Verification items for the finished model (mm, model axes). Face numbers are marked on the shaded views. Round coordinates to 2 decimals unless told otherwise and drop trailing zeros. Loops run counter-clockwise (first coordinate to the right, second up) from the corner with the lowest first, then second, coordinate; pieces in that order, holes last. Notation, with made-up numbers: M 49,19.5 L 59,19.5 A14 ccw 59,34.5 Z; hole C -32.5,-38 d9. An arc over 180 degrees is marked long. Answer as CSV lines item,"result".
Autodesk Inventor part; units mm, degrees
ref_plane "Work Plane1" through (0, 5, 0) normal (0, 1, 0) x (1, 0, 0)
ref_plane "Work Plane2" through (0, 0, 0) normal (0, -1, 0) x (1, 0, 0)
ref_plane "YZ Plane" through (0, 0, 0) normal (1, 0, 0) x (0, 1, 0)
sketch "Sketch1" plane through (0, 0, 0) normal (0, 1, 0) x (-1, 0, 0)
  line L0 (2.8251, -4.9022) -> (-2.8329, -4.8978)
  line L1 (-2.8329, -4.8978) -> (-5.658, 0.0045)
  line L2 (-5.658, 0.0045) -> (-2.8251, 4.9022)
  line L3 (-2.8251, 4.9022) -> (2.8329, 4.8978)
  line L4 (2.8329, 4.8978) -> (5.658, -0.0045)
  line L5 (5.658, -0.0045) -> (2.8251, -4.9022)
  circle A0 centre (0, 0) radius 3
  dimension "d0" = 9.8
  dimension "d1" = 6
extrude "Extrusion1" add sketch "Sketch1" along normal blind 5
fillet "Fillet1" radius 0.8 14 edges at (4.2416, 5, 2.4533) (4.2455, 5, -2.4467) (0.0039, 5, -4.9) (-4.2416, 5, -2.4533) (-4.2455, 5, 2.4467) (-0.0039, 5, 4.9) (-0.0039, 0, 4.9) (4.2416, 0, 2.4533) (4.2455, 0, -2.4467) (0.0039, 0, -4.9) (-4.2416, 0, -2.4533) (-4.2455, 0, 2.4467) (3, 5, 0) (3, 0, 0)
thread "Thread1"
ref_plane "Work Plane1" through (0, 5, 0) normal (0, 1, 0) x (1, 0, 0)
ref_plane "Work Plane2" through (0, 0, 0) normal (0, -1, 0) x (1, 0, 0)
properties part number "m6nut"
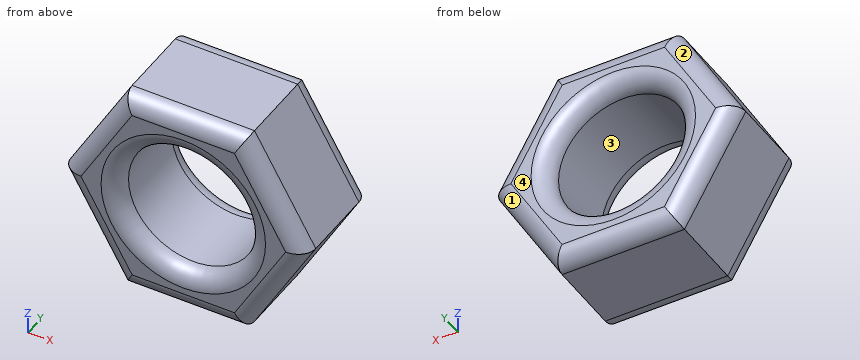
1) Section check A-A (y = 2.8). Record the cut outline in (x, z).
Here are the results:
outline,"M -5.66,0 L -2.83,-4.9 L 2.83,-4.9 L 5.66,0 L 2.83,4.9 L -2.83,4.9 Z; hole C 0,0 d6"
2) Go/stop test with flat-tipped pins: pin 1 (2 mm diameter, centred on y = 1, z = -3.5, fed in from -X); pin 2 (5.5 mm diameter, centred on x = 0, z = 0, fed in from +Y); pin 3 (1 mm diameter, centred on x = 4, z = -0.5, fed in from -Y); pin 4 (1 mm diameter, centred on x = -1, y = 1.5, fed in from +Z). Record where each tip stops, or that it passes through.
Here are the results:
pin 1,"stops at x = -4.21"
pin 2,"passes through"
pin 3,"stops at y = 0"
pin 4,"stops at z = 4.9"
3) Section check B-B (y = 0.5). Record the cut outline in (x, z).
Here are the results:
outline,"M -5.59,0 L -2.79,-4.84 L 2.8,-4.84 L 5.59,0 L 2.79,4.84 L -2.8,4.84 Z; hole C 0,0 d6.12"
4) Draft check along Z on the marked faces 1, 2, 3 and 4. Enter one of: +Z half, -Z half, draft (parallel to the pull), parting line (faces both ways), or undercut.
Here are the results:
face 1,"-Z half"
face 2,"+Z half"
face 3,"undercut"
face 4,"draft"
5) Material ranges on probe 1 along Z at (x, y) = (0, 2.55); probe 2 along X at (y, z) = (3.5, -2.5); probe 3 along X at (y, z) = (4.1, 2.75), recorded low to high.
Here are the results:
probe 1,"z = -4.9 to -3, 3 to 4.9"
probe 2,"x = -4.21 to -1.66, 1.66 to 4.21"
probe 3,"x = -4.07 to -1.2, 1.2 to 4.07"
